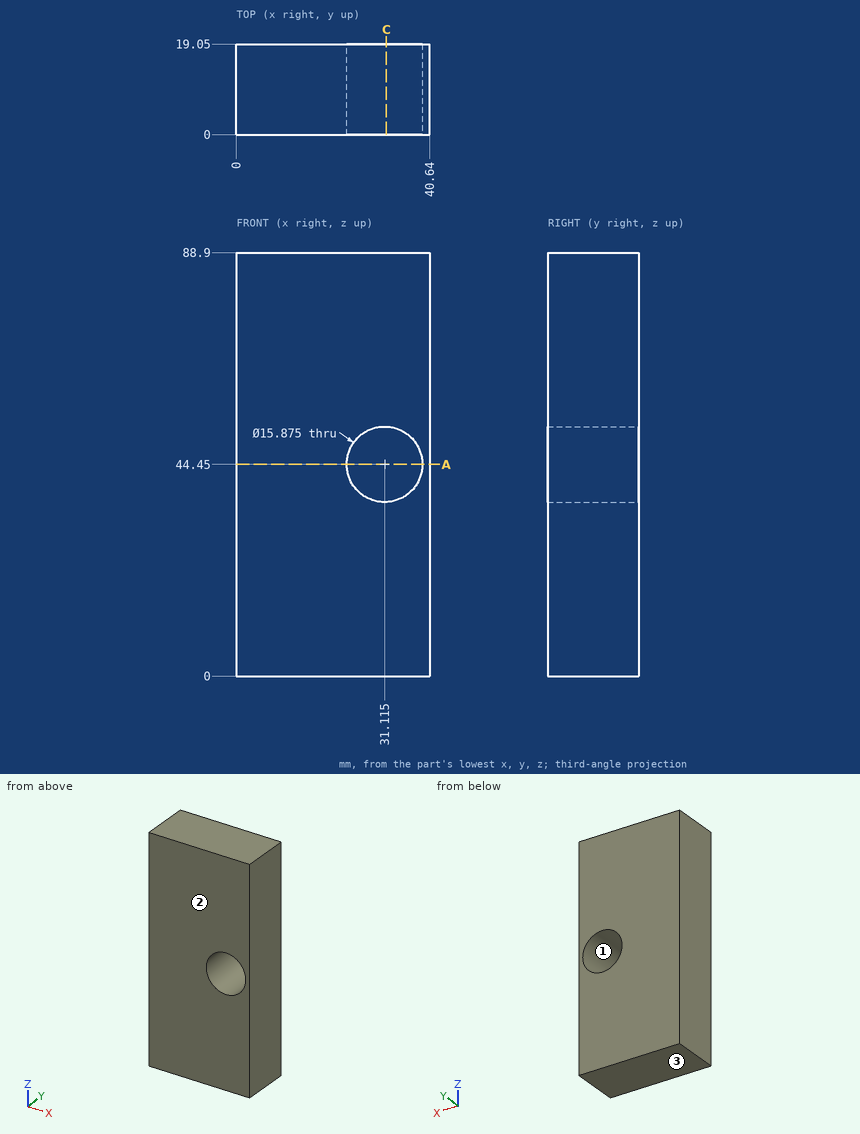
Design review of the part shown in the three views and the two pictorial views. Dimensions are in mm from the part's minimum x, y and z. Coordinates: 2 decimals unless noted, no trailing zeros. Order: outer loops, then holes, each group sorted by start corner. A loop starts at its lowest first (then second) coordinate and runs counter-clockwise, first axis right, second up. Notation, with made-up numbers: (30, 48.5) -> (45, 48.5) arc R18 cw to (45, 83.5) -> close; hole circle Ø8 at (-2.5, 46). An arc over 180 degrees is marked (long way). Use one line per item in the form item = value. Start each with the question number.
(1) For probe 1 along Z at (x, y) = (31.5, 9); probe 2 along X at (y, z) = (12.5, 44.45); probe 3 along X at (y, z) = (2, 50.5), list the stretches that pass through material, from the lowest coordinate up.
(2) Add section A-A on z = 44.45. State the section outline as (x, y) points, plus the area to 3 significant figures.
(3) Add section C-C on x = 31.5. State the section outline as (y, z) points.
(4) Insertion check: pin 1 (1.5 mm diameter, centred on y = 5.5, z = 23, fed in from -X). The pin has a flat end and moves straight along its axis. Give the tip position at first contact, or say it passes through.
(5) The part is to be moulded in two halves that separate along Z. For the marked faces 1, 2 and 3, say which applies: +Z half, -Z half, draft (parallel to the pull), parting line (faces both ways), or undercut.
Answer block:
q1.probe_1 = 0 to 36.52, 52.38 to 88.9
q1.probe_2 = 0 to 23.18, 39.05 to 40.64
q1.probe_3 = 0 to 25.98, 36.25 to 40.64
q2.outline = (0, 0) -> (23.18, 0) -> (23.18, 19.05) -> (0, 19.05) -> close; (39.05, 0) -> (40.64, 0) -> (40.64, 19.05) -> (39.05, 19.05) -> close
q2.area = 472 mm²
q3.outline = (0, 0) -> (19.05, 0) -> (19.05, 36.52) -> (0, 36.52) -> close; (0, 52.38) -> (19.05, 52.38) -> (19.05, 88.9) -> (0, 88.9) -> close
q4.pin_1 = 0
q5.face_1 = undercut
q5.face_2 = draft
q5.face_3 = -Z half
